from build123d import *

# Parameters (mm, degrees)
BOSS_EXTRUDE1_DEPTH = 1000
CUT_EXTRUDE1_DEPTH  = 5
FILLET1_R           = 2


with BuildPart() as part:
    # Sketch1 → Boss-Extrude1 (new body)
    with BuildSketch(Plane(origin=(0, 0, 0), x_dir=(0, 0, -1), z_dir=(1, 0, 0))):
        with BuildLine():
            Line((-21.263810414, 3.81), (-5.08, 31.841181898))
            ThreePointArc((-5.08, 31.841181898), (0, 50.8), (5.08, 31.841181898))
            Line((5.08, 31.841181898), (21.263810414, 3.81))
            Line((21.263810414, 3.81), (26.343810414, 3.81))
            Line((26.343810414, 3.81), (26.343810414, 5.588))
            Line((26.343810414, 5.588), (31.75, 5.588))
            Line((31.75, 5.588), (31.75, 0))
            Line((31.75, 0), (-31.75, 0))
            Line((-31.75, 0), (-31.75, 5.588))
            Line((-31.75, 5.588), (-26.343810414, 5.588))
            Line((-26.343810414, 5.588), (-26.343810414, 3.81))
            Line((-26.343810414, 3.81), (-21.263810414, 3.81))
        make_face()
    extrude(amount=BOSS_EXTRUDE1_DEPTH)

    # Sketch2 → Cut-Extrude1 (cut)
    with BuildSketch(Plane.ZY):
        with BuildLine():
            Line((19.999413325, 0), (18.267362517, 3))
            Line((18.267362517, 3), (3.808670233, 28.043189647))
            ThreePointArc((3.808670233, 28.043189647), (0, 27.48), (-3.808670233, 28.043189647))
            Line((-3.808670233, 28.043189647), (-18.267362517, 3))
            Line((-18.267362517, 3), (-19.999413325, 0))
            Line((-19.999413325, 0), (19.999413325, 0))
        make_face()
    cut_extrude1 = extrude(amount=-CUT_EXTRUDE1_DEPTH, mode=Mode.SUBTRACT)

    # Mirror1: Cut-Extrude1 across plane
    add(cut_extrude1.mirror(Plane.ZY.offset(-500)), mode=Mode.SUBTRACT)

    # Fillet1
    # the kernel refuses this fillet: 2 mm, written as the material it takes off along each edge
    with BuildSketch(Plane(origin=(-5, 0, 31.75), x_dir=(0, 1, 0), z_dir=(1, 0, 0)), Plane(origin=(-5, 5.588, 31.75), x_dir=(0, 0, -1), z_dir=(1, 0, 0)), Plane(origin=(-5, 0, -31.75), x_dir=(0, 0, 1), z_dir=(1, 0, 0)), Plane(origin=(-5, 5.588, -31.75), x_dir=(0, -1, 0), z_dir=(1, 0, 0))) as fillet1_piece_1:
        with BuildLine():
            CenterArc((FILLET1_R, -FILLET1_R), FILLET1_R, 90, 90)
            Line((0, -FILLET1_R), (-FILLET1_R * 0.02, -FILLET1_R))
            Line((-FILLET1_R * 0.02, -FILLET1_R), (-FILLET1_R * 0.02, FILLET1_R * 0.02))
            Line((-FILLET1_R * 0.02, FILLET1_R * 0.02), (FILLET1_R, FILLET1_R * 0.02))
            Line((FILLET1_R, FILLET1_R * 0.02), (FILLET1_R, 0))
        make_face()
    extrude(amount=1010, mode=Mode.SUBTRACT)
    with BuildSketch(Plane(origin=(-4.969102032, 5.588, 26.343810414), x_dir=(0, -1, 0), z_dir=(1, 0, 0))) as fillet1_piece_2:
        with BuildLine():
            CenterArc((2, -1.987640813), FILLET1_R, 96.372964386, 83.627035614)
            Line((0, -1.987640813), (-0.04, -1.987640813))
            Line((-0.04, -1.987640813), (-0.04, 0))
            Line((-0.04, 0), (0, 0.04))
            ThreePointArc((0, 0.04), (0.889, 0.04), (1.77356, 0.039752816))
            Line((1.77356, 0.039752816), (1.778, 0))
        make_face()
    extrude(amount=1009.938204063, mode=Mode.SUBTRACT)
    with BuildSketch(Plane(origin=(-4.969102032, 5.588, -26.343810414), x_dir=(0, 0, -1), z_dir=(1, 0, 0))) as fillet1_piece_3:
        with BuildLine():
            CenterArc((1.987640813, -2), FILLET1_R, 90, 83.627035614)
            Line((0, -1.778), (-0.039752816, -1.77356))
            ThreePointArc((-0.039752816, -1.77356), (-0.04, -0.889), (-0.04, 0))
            Line((-0.04, 0), (0, 0.04))
            Line((0, 0.04), (1.987640813, 0.04))
            Line((1.987640813, 0.04), (1.987640813, 0))
        make_face()
    extrude(amount=1009.938204063, mode=Mode.SUBTRACT)


solid = part.part
For this review, take the finished solid that the model builds, in its own axes (mm). Round coordinates to 2 decimals unless told otherwise and drop trailing zeros. Write each loop counter-clockwise with the first axis right and the second up, starting at its lowest first coordinate (ties: lowest second). Pieces come first, ordered by that corner, then holes. Notation, with made-up numbers: (67.5, 57) -> (112.5, 57) arc R34 ccw to (112.5, 88) -> close; hole circle Ø10 at (-30.5, 86.5). An arc over 180 degrees is marked (long way). Use CSV: the item, a comma, the result in double quotes.
(1) Draft analysis for pull direction Z (two halves, no side actions). For faces 1 (the face through (493, 50.793, 0.372)), 2 (the face through (5, 11, 0)), 3 (the face through (995, 11, 0)), 4 (the face through (493, 0, 0)), state which applies: +Z half, -Z half, draft (parallel to the pull), parting line (faces both ways), or undercut.
Computed values:
face 1,"parting line"
face 2,"undercut"
face 3,"undercut"
face 4,"draft"
(2) To check wall thickness, follow L1, parallel to Z at x = 248.5, y = 4; L2, parallel to Y at x = 559.5, z = -27.5; L3, parallel to X at y = 13, z = 10.5. State the ranges of each line that lie inside material, in increasing order. Write a range as [from, to].
Computed values:
L1,"[-31.71, -26.37], [-21.15, 21.15], [26.37, 31.71]"
L2,"[0, 5.41]"
L3,"[5, 995]"
(3) Consider section B-B, the plane y = 40.64. Give the boundary of the cut face in (x, z), plus the area to 3 significant figures.
Computed values:
outline,"(0, -10.16) -> (1000, -10.16) -> (1000, 10.16) -> (0, 10.16) -> close"
area,"20,300 mm²"
(4) Consider section A-A, the plane x = 746.5. Give the boundary of the cut face in (y, z).
Computed values:
outline,"(0, -29.75) arc R2 ccw to (2, -31.75) -> (3.59, -31.75) arc R2 ccw to (5.59, -29.75) -> (5.59, -28.33) arc R2 ccw to (3.81, -26.34) -> (3.81, -21.26) -> (31.84, -5.08) arc R10.16 ccw (long way) to (31.84, 5.08) -> (3.81, 21.26) -> (3.81, 26.34) arc R2 ccw to (5.59, 28.33) -> (5.59, 29.75) arc R2 ccw to (3.59, 31.75) -> (2, 31.75) arc R2 ccw to (0, 29.75) -> close"
(5) Clearance check with flat-ended pins moving along their axes: P1, Ø1.5, axis at x = 200, z = 5, coming from the +Y side; P2, Ø5, axis at y = 5.5, z = -0.5, coming from the -X side; P3, Ø4, axis at x = 158, z = 21.5, coming from the +Y side (3 decimals). State where each tip first meets the part, or that it passes through.
Computed values:
P1,"y = 49.87"
P2,"x = 5"
P3,"y = 6.865"
